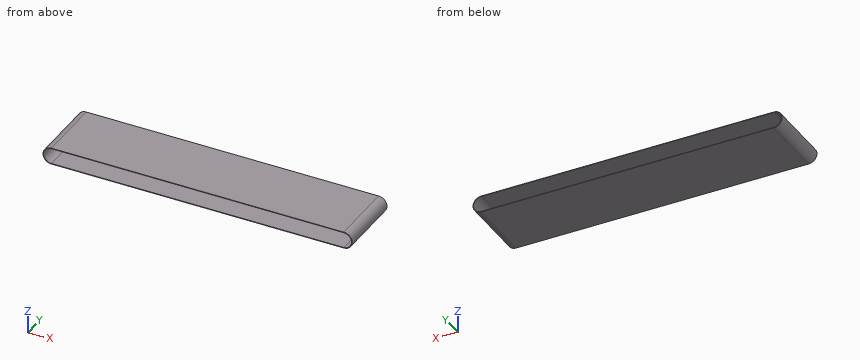
Autodesk Inventor part; units mm, degrees
ref_plane "YZ Plane" through (0, 0, 0) normal (1, 0, 0) x (0, 1, 0)
ref_plane "XZ Plane" through (0, 0, 0) normal (0, 1, 0) x (-1, 0, 0)
ref_plane "XY Plane" through (0, 0, 0) normal (0, 0, 1) x (1, 0, 0)
sketch "Skizze1" plane through (0, 0, 0) normal (0, 1, 0) x (-1, 0, 0)
  arc A0 (0, -40) -> (0, 40) centre (0, 0) ccw
  arc A1 (0, -43) -> (0, 43) centre (0, 0) ccw
  arc A2 (-1500, 40) -> (-1500, -40) centre (-1500, 0) ccw
  arc A3 (-1500, 43) -> (-1500, -43) centre (-1500, 0) ccw
  line L0 (0, 43) -> (-1500, 43)
  line L1 (-1500, 40) -> (0, 40)
  line L2 (0, -40) -> (-1500, -40)
  line L3 (-1500, -43) -> (0, -43)
  dimension "d0" = 80
  dimension "d1" = 86
  dimension "d2" = 80
  dimension "d3" = 86
  dimension "d4" = 1500
extrude "Extrusion1" add sketch "Skizze1" along normal blind 340
properties part number "Band"
CAD build for the part. Positions are in the model's coordinates, mm. Coordinates: 2 decimals unless noted, no trailing zeros. Order: outer loops, then holes, each group sorted by start corner. A loop starts at its lowest first (then second) coordinate and runs counter-clockwise, first axis right, second up. Notation, with made-up numbers: (7, 60.25) -> (31, 60.25) arc R33 ccw to (31, 92.25) -> close; hole circle Ø7 at (54, 82.25). An arc over 180 degrees is marked (long way). Use one line per item in the form item = value. Start each with the question number.
1) Band-saw the part on A-A on y = 256. Give the cut face in (x, z).
2) Band-saw the part on B-B on x = 1121.5. Give the cut face in (y, z).
3) Band-saw the part on C-C on z = 0. Give the cut face in (x, y).
4) Drop flat-ended pins along their axis: pin 1 (8 mm diameter, centred on y = 266.5, z = -8.5, fed in from +X); pin 2 (2 mm diameter, centred on y = 210.5, z = 21.5, fed in from +X); pin 3 (6 mm diameter, centred on y = 80.5, z = -14.5, fed in from -X). Give the stop position or say it passes through.
5) Drill centre lines: L1, parallel to Z at x = 1389, y = 130; L2, parallel to X at y = 18.5, z = 3.5; L3, parallel to X at y = 101.5, z = -24. Where is each one in solid material? Low to high. Write a range as [from, to].
Entries:
q1.outline = (0, -43) -> (1500, -43) arc R43 ccw to (1500, 43) -> (0, 43) arc R43 ccw to start; hole (0, -40) -> (1500, -40) arc R40 ccw to (1500, 40) -> (0, 40) arc R40 ccw to start
q2.outline = (0, -43) -> (340, -43) -> (340, -40) -> (0, -40) -> close; (0, 40) -> (340, 40) -> (340, 43) -> (0, 43) -> close
q3.outline = (-43, 0) -> (-40, 0) -> (-40, 340) -> (-43, 340) -> close; (1540, 0) -> (1543, 0) -> (1543, 340) -> (1540, 340) -> close
q4.pin_1 = 1542.76
q4.pin_2 = 1537.8
q4.pin_3 = -41.43
q5.L1 = [-43, -40], [40, 43]
q5.L2 = [-42.86, -39.85], [1539.85, 1542.86]
q5.L3 = [-35.68, -32], [1532, 1535.68]
